Model file for the job. Use its own axes, mm. A direction names the side the tool comes from. Give positions to 0.01 mm unless a question says otherwise; leave off trailing zeros. Write each loop counter-clockwise with the first axis right and the second up, starting at its lowest first coordinate (ties: lowest second). Pieces come first, ordered by that corner, then holes.
```python
from build123d import *

# Parameters (mm, degrees)
Y_KSEKLIK_EKSTR_ZYON1_DEPTH      = 15
Y_KSEKLIK_EKSTR_ZYON1_DEPTH_BACK = 15
KES_EKSTR_ZYON2_START            = -10
IZIM1_8_R                        = 27.5
IZIM1_8_R_2                      = 21.5
KES_EKSTR_ZYON2_DEPTH            = 39
IZIM1_11_R                       = 21.5
IZIM1_11_R_2                     = 17
Y_KSEKLIK_EKSTR_ZYON4_DEPTH      = 30
KES_EKSTR_ZYON3_DEPTH            = 26
KES_EKSTR_ZYON3_DEPTH_BACK       = 47
IZIM1_12_R                       = 17
KES_EKSTR_ZYON4_DEPTH            = 47
KES_EKSTR_ZYON4_DEPTH_BACK       = 47
IZIM1_13_R                       = 10


with BuildPart() as part:
    # izim1 → Y_kseklik-Ekstr_zyon1 (new, two sides: drawn at the far end of the back side and taken through both)
    with BuildSketch(Plane.XY.offset(-Y_KSEKLIK_EKSTR_ZYON1_DEPTH_BACK)):
        with BuildLine():
            ThreePointArc((-26.678302647, -12.37237703), (0, -62.043488141), (26.678302647, -12.37237703))
            ThreePointArc((26.678302647, -12.37237703), (16.836772686, 12.870553113), (18.321243986, 39.923419489))
            ThreePointArc((18.321243986, 39.923419489), (0, 63.956511859), (-18.321243986, 39.923419489))
            ThreePointArc((-18.321243986, 39.923419489), (-16.836772686, 12.870553113), (-26.678302647, -12.37237703))
        make_face()
    extrude(amount=Y_KSEKLIK_EKSTR_ZYON1_DEPTH + Y_KSEKLIK_EKSTR_ZYON1_DEPTH_BACK)

    # izim1_8 → Kes-Ekstr_zyon2 (cut)
    with BuildSketch(Plane.XY.offset(KES_EKSTR_ZYON2_START)):
        with Locations((0, -30.043488141)):
            Circle(IZIM1_8_R)
        with Locations((0, -30.043488141)):
            Circle(IZIM1_8_R_2, mode=Mode.SUBTRACT)
    extrude(amount=-KES_EKSTR_ZYON2_DEPTH, mode=Mode.SUBTRACT)

    # izim1_11 → Y_kseklik-Ekstr_zyon4 (add)
    # profile 1 of 2: a face of its own
    with BuildSketch(Plane.XY):
        with Locations((0, -30.043488141)):
            Circle(IZIM1_11_R)
        with Locations((0, -30.043488141)):
            Circle(IZIM1_11_R_2, mode=Mode.SUBTRACT)
    # profile 2 of 2: a face of its own
    with BuildSketch(Plane.XY):
        with Locations((0, -30.043488141)):
            Circle(IZIM1_11_R_2)
    extrude(amount=-Y_KSEKLIK_EKSTR_ZYON4_DEPTH)

    # izim1_12 → Kes-Ekstr_zyon3 (cut, two sides: drawn at the far end of the back side and taken through both)
    with BuildSketch(Plane.XY.offset(-KES_EKSTR_ZYON3_DEPTH_BACK)):
        with Locations((0, -30.043488141)):
            Circle(IZIM1_12_R)
    extrude(amount=KES_EKSTR_ZYON3_DEPTH + KES_EKSTR_ZYON3_DEPTH_BACK, mode=Mode.SUBTRACT)

    # izim1_13 → Kes-Ekstr_zyon4 (cut, two sides: drawn at the far end of the back side and taken through both)
    with BuildSketch(Plane.XY.offset(-KES_EKSTR_ZYON4_DEPTH_BACK)):
        with Locations((0, 44.956511859)):
            Circle(IZIM1_13_R)
    extrude(amount=KES_EKSTR_ZYON4_DEPTH + KES_EKSTR_ZYON4_DEPTH_BACK, mode=Mode.SUBTRACT)


solid = part.part
```
1. Slice it at C-C, the plane z = 3. Write the cut outline in (x, y).
Calculated:
outline: (-26.68, -12.37) arc R32 ccw (long way) to (26.68, -12.37) arc R64 cw to (18.32, 39.92) arc R19 ccw (long way) to (-18.32, 39.92) arc R64 cw to start; hole circle Ø34 at (0, -30.04); hole circle Ø20 at (0, 44.96)
2. Pin check, flat tips, straight feed: P1, Ø12, axis at x = 4.5, z = 3.5, coming from the +Y side; P2, Ø10, axis at x = -6, z = 2.5, coming from the +Y side; P3, Ø1, axis at y = -36.5, z = -18.5, coming from the -X side. Stop position of each tip, or through.
Calculated:
P1: stops at y = 63.96
P2: stops at y = 63.93
P3: stops at x = -20.66
3. Which spindle directions (+Z, -Z, +X, -X, +Y, -Y) get a long thin tool onto all of the face, cutting with end or side? Do faces 4 (the cylindrical face through (-1.3, 54.87, -0.21)), 5 (the cylindrical face through (12.69, -54.44, -12.46)). Say none if no direction does.
Calculated:
face 4: +Z, -Z
face 5: -Z
4. Slice it at A-A, the plane x = 0. Write the cut outline in (y, z), and give its area (4 significant figures).
Calculated:
outline: (-62.04, -15) - (-57.54, -15) - (-57.54, -10) - (-51.54, -10) - (-51.54, -30) - (-47.04, -30) - (-47.04, 15) - (-62.04, 15) - close; (-13.04, -30) - (-8.54, -30) - (-8.54, -10) - (-2.54, -10) - (-2.54, -15) - (34.96, -15) - (34.96, 15) - (-13.04, 15) - close; (54.96, -15) - (63.96, -15) - (63.96, 15) - (54.96, 15) - close
area: 2,235 mm2
5. Probe probe 1 along Y at (x, z) = (-13, -10.5); probe 2 along Y at (x, z) = (-4, 1); probe 3 along Y at (x, z) = (-1, -14). List the from-to ranges inside material, lowest first.
Calculated:
probe 1: y = -59.28 to -54.28, -47.17 to -41, -19.09 to -12.92, -5.81 to 58.81
probe 2: y = -61.79 to -46.57, -13.52 to 35.79, 54.12 to 63.53
probe 3: y = -62.03 to -57.53, -51.52 to -47.01, -13.07 to -8.57, -2.56 to 35.01, 54.91 to 63.93
6. Slice it at B-B, the plane y = -21. Write the cut outline in (x, z), and give its area (3 significant figures).
Calculated:
outline: (-30.7, -15) - (-25.97, -15) - (-25.97, -10) - (-19.51, -10) - (-19.51, -30) - (-14.39, -30) - (-14.39, 15) - (-30.7, 15) - close; (14.39, -30) - (19.51, -30) - (19.51, -10) - (25.97, -10) - (25.97, -15) - (30.7, -15) - (30.7, 15) - (14.39, 15) - close
area: 1,070 mm2
7. Slice it at D-D, the plane y = -45. Write the cut outline in (x, z).
Calculated:
outline: (-28.29, -15) - (-23.08, -15) - (-23.08, -10) - (-15.45, -10) - (-15.45, -30) - (-8.08, -30) - (-8.08, 15) - (-28.29, 15) - close; (8.08, -30) - (15.45, -30) - (15.45, -10) - (23.08, -10) - (23.08, -15) - (28.29, -15) - (28.29, 15) - (8.08, 15) - close
8. Pull direction Y, two halves, no side cores. Call faces 1 (the cylindrical face through (-0.97, -62.03, -0.21)), 2 (the cylindrical face through (-4.661, -51.032, -19.86)), 3 (the flat face through (0, 6, -15)): +Y half, -Y half, draft (parallel to the pull), parting line (faces both ways), or undercut.
Calculated:
face 1: parting line
face 2: undercut
face 3: draft
